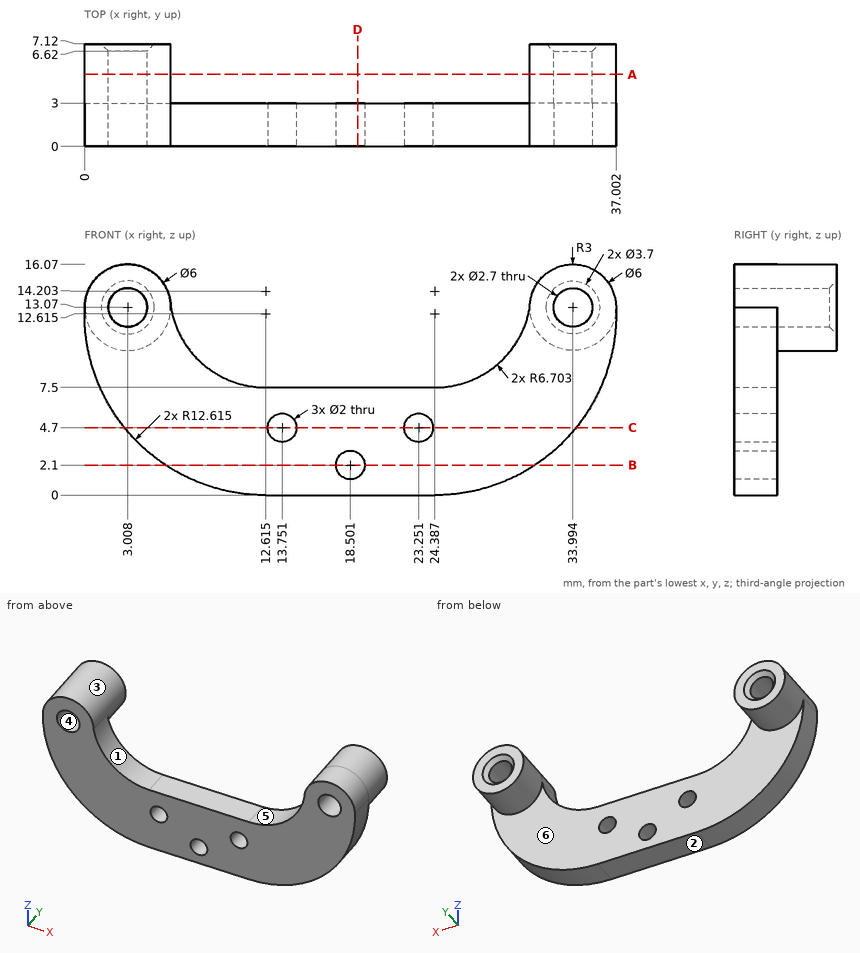
For this review, use the dimensioned drawing (mm, ordinates from the lowest corner) and the shaded views. A direction names the side the tool comes from. Round coordinates to 2 decimals unless told otherwise and drop trailing zeros. Write each loop counter-clockwise with the first axis right and the second up, starting at its lowest first coordinate (ties: lowest second). Pieces come first, ordered by that corner, then holes. Notation, with made-up numbers: (10.25, 26.5) - (20.25, 26.5) arc R7 ccw to (20.25, 31.5) - close; hole circle Ø9 at (-37, -16.75). An arc over 180 degrees is marked (long way). Use CSV: the item, a comma, the result in double quotes.
1) Add section D-D on x = 19. Write out the cut boundary in (y, z).
Conclusion:
outline,"(0, 0) - (3, 0) - (3, 1.23) - (0, 1.23) - close; (0, 2.97) - (3, 2.97) - (3, 7.5) - (0, 7.5) - close"
2) Clearance check with flat-ended pins moving along their axes: pin 1 Ø3 at (y, z) = (2, 4.5) entering from -X; pin 2 Ø1.5 at (y, z) = (1.5, 5) entering from +X; pin 3 Ø1.5 at (x, y) = (17.5, 1) entering from +Z. State where each tip first meets the part, or that it passes through.
Conclusion:
pin 1,"stops at x = 1.87"
pin 2,"stops at x = 34.97"
pin 3,"stops at z = 7.5"
3) Add section A-A on y = 5. Write out the cut boundary in (x, z), and give its area (3 significant figures).
Conclusion:
outline,"circle Ø6 at (3.01, 13.07); circle Ø6 at (33.99, 13.07); hole circle Ø2.7 at (3.01, 13.07); hole circle Ø2.7 at (33.99, 13.07)"
area,"45.1 mm^2"
4) For the marked faces 1 and 2, list the 3-axis set-ups (+Z, -Z, +X, -X, +Y, -Y) from which the entire face can be reached by the end or side of a thin tool; tool diameter is ignored.
Conclusion:
face 1,"+Z, +Y, -Y"
face 2,"-Z, +X, -X, +Y, -Y"
5) The part is to be moulded in two halves that separate along Z. For the marked faces 3, 4, 5 and 6, say which applies: pulls with the +Z half, pulls with the -Z half, needs draft (parallel to the pull), parting line crosses it, or undercut.
Conclusion:
face 3,"parting line crosses it"
face 4,"undercut"
face 5,"pulls with the +Z half"
face 6,"needs draft"
6) Add section C-C on z = 4.7. Write out the cut boundary in (x, y).
Conclusion:
outline,"(2.79, 0) - (12.75, 0) - (12.75, 3) - (2.79, 3) - close; (14.75, 0) - (22.25, 0) - (22.25, 3) - (14.75, 3) - close; (24.25, 0) - (34.21, 0) - (34.21, 3) - (24.25, 3) - close"
7) Wall thickness on line 1 along X through (y, z) = (1.05, 4.7); line 2 along Y through (x, z) = (27.5, 8); line 3 along X through (y, z) = (6.75, 14.75): over which ranges is each line inside the solid? List them lowest first. Write a range as from..to.
Conclusion:
line 1,"x = 2.79..12.75, 14.75..22.25, 24.25..34.21"
line 2,"y = 0..3"
line 3,"x = 0.52..5.49, 31.51..36.48"
8) Add section B-B on z = 2.1. Write out the cut boundary in (x, y) (1 decimal).
Conclusion:
outline,"(5.6, 0) - (17.5, 0) - (17.5, 3) - (5.6, 3) - close; (19.5, 0) - (31.4, 0) - (31.4, 3) - (19.5, 3) - close"
